For this review, use the dimensioned drawing (mm, ordinates from the lowest corner) and the shaded views. A direction names the side the tool comes from. Round coordinates to 2 decimals unless told otherwise and drop trailing zeros. Write each loop counter-clockwise with the first axis right and the second up, starting at its lowest first coordinate (ties: lowest second). Pieces come first, ordered by that corner, then holes. Notation, with made-up numbers: (-8, 64.25) - (1, 64.25) arc R28 cw to (1, 92.25) - close; hole circle Ø6 at (11.5, 21). An arc over 180 degrees is marked (long way). Write each question's results on one line, items separated by ' | '.
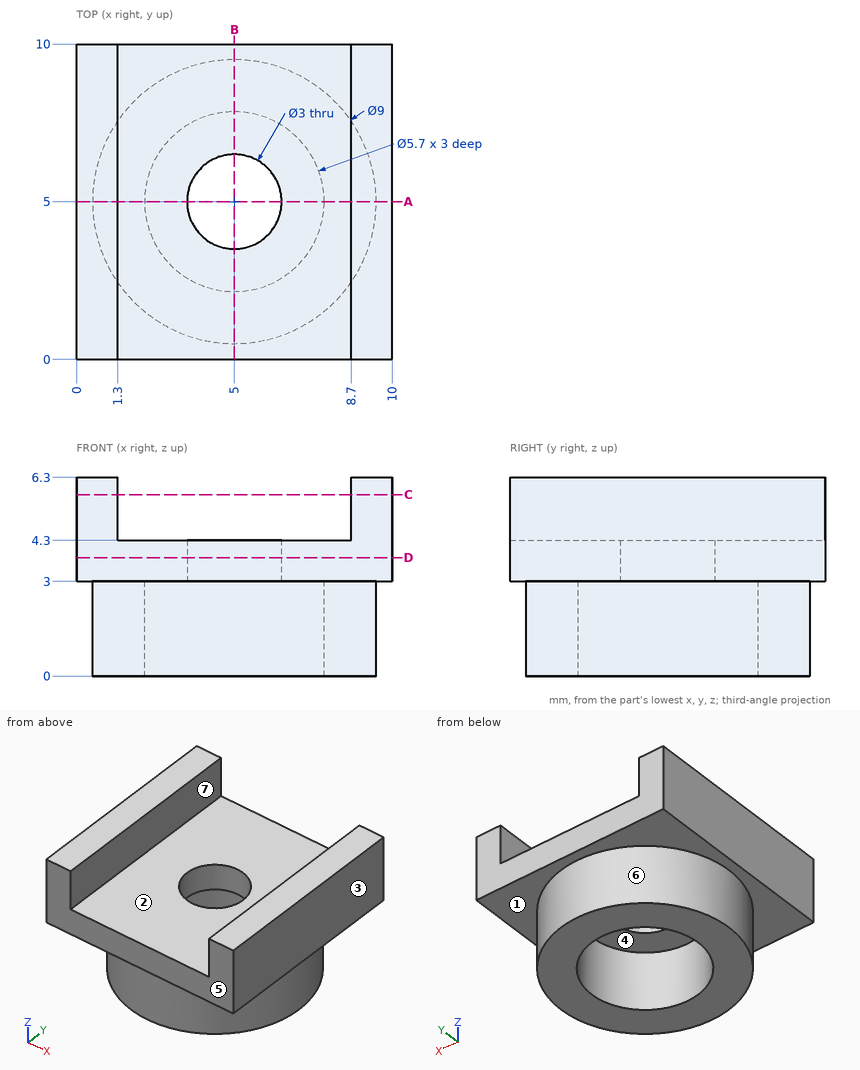
Q1. We need section D-D (z = 3.75). State the section outline as (x, y) points, plus the area to 3 significant figures.
Evaluation:
outline: (0, 0) - (10, 0) - (10, 10) - (0, 10) - close; hole circle Ø3 at (5, 5) | area: 92.9 mm^2
Q2. For probe 1 along Y at (x, z) = (5, 3.5); probe 2 along X at (y, z) = (7.75, 5.25); probe 3 along Z at (x, y) = (7.75, 7.25), list the stretches that pass through material, from the lowest coordinate up.
Evaluation:
probe 1: y = 0 to 3.5, 6.5 to 10 | probe 2: x = 0 to 1.3, 8.7 to 10 | probe 3: z = 0 to 4.3
Q3. We need section A-A (y = 5). State the section outline as (x, z) points.
Evaluation:
outline: (0, 3) - (0.5, 3) - (0.5, 0) - (2.15, 0) - (2.15, 3) - (3.5, 3) - (3.5, 4.3) - (1.3, 4.3) - (1.3, 6.3) - (0, 6.3) - close; (6.5, 3) - (7.85, 3) - (7.85, 0) - (9.5, 0) - (9.5, 3) - (10, 3) - (10, 6.3) - (8.7, 6.3) - (8.7, 4.3) - (6.5, 4.3) - close
Q4. Insertion check: P1, Ø1.5, axis at x = 6, y = 8.5, coming from the +Z side; P2, Ø4, axis at x = 3.5, y = 1.5, coming from the -Z side; P3, Ø2, axis at x = 7, z = 1, coming from the -Y side; P4, Ø1.7, axis at x = 4, y = 4, coming from the -Z side. Each pin has a flat end and moves straight along its axis. Give the tip position at first contact, or say it passes through.
Evaluation:
P1: stops at z = 4.3 | P2: stops at z = 0 | P3: stops at y = 0.61 | P4: stops at z = 3
Q5. The part is to be moulded in two halves that separate along Y. For the marked faces 4, 5, 6 and 7, say which applies: released by +Y, released by -Y, zero draft, split by the parting line, or undercut.
Evaluation:
face 4: undercut | face 5: released by -Y | face 6: split by the parting line | face 7: zero draft
Q6. Tool access review of the marked faces 1, 2 and 3: name each direction out of +Z, -Z, +X, -X, +Y, -Y from which nothing blocks a thin tool from reaching the whole face with its end or side.
Evaluation:
face 1: -Z | face 2: +Z, +Y, -Y | face 3: +Z, -Z, +X, +Y, -Y
Q7. We need section B-B (x = 5). State the section outline as (y, z) points, plus the area to 3 significant figures.
Evaluation:
outline: (0, 3) - (0.5, 3) - (0.5, 0) - (2.15, 0) - (2.15, 3) - (3.5, 3) - (3.5, 4.3) - (0, 4.3) - close; (6.5, 3) - (7.85, 3) - (7.85, 0) - (9.5, 0) - (9.5, 3) - (10, 3) - (10, 4.3) - (6.5, 4.3) - close | area: 19.0 mm^2
Q8. We need section C-C (z = 5.75). State the section outline as (x, y) points.
Evaluation:
outline: (0, 0) - (1.3, 0) - (1.3, 10) - (0, 10) - close; (8.7, 0) - (10, 0) - (10, 10) - (8.7, 10) - close
